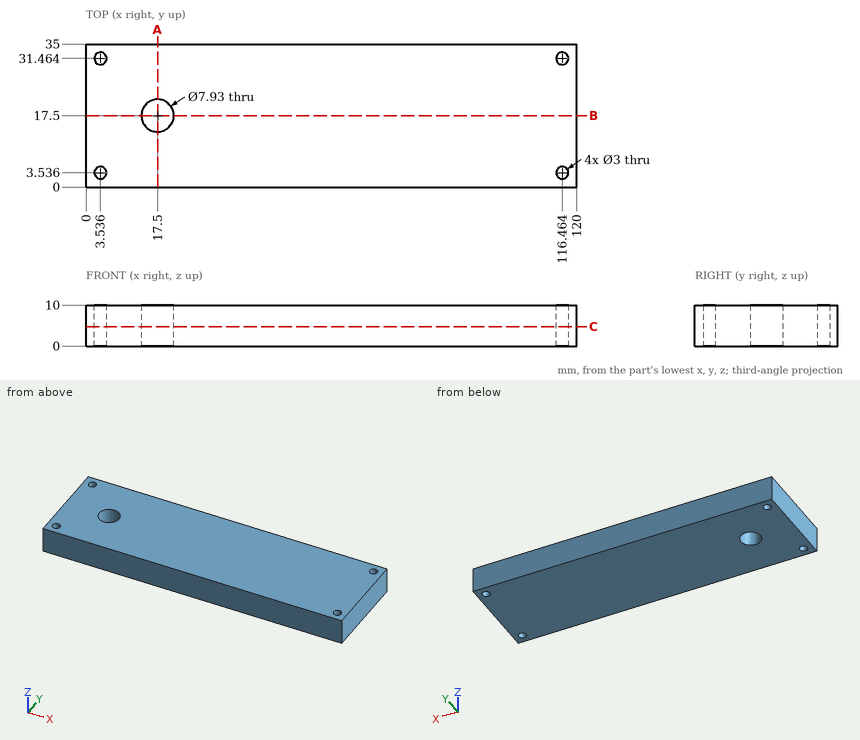
Verification items for this drawing (mm, ordinates from the low corner). Give positions to 0.01 mm unless a question says otherwise; leave off trailing zeros. Write each loop counter-clockwise with the first axis right and the second up, starting at its lowest first coordinate (ties: lowest second). Pieces come first, ordered by that corner, then holes. Notation, with made-up numbers: (13, 26) - (64, 26) arc R21 cw to (64, 33) - close; hole circle Ø3 at (47, 28.5). An arc over 180 degrees is marked (long way). Answer as a JSON object with one key per item and string values. Group by question number.
1) Sectioned sample at A-A (x = 17.5). Record the cut outline in (y, z) (1 decimal).
2) Sectioned sample at B-B (y = 17.5). Record the cut outline in (x, z) (1 decimal).
3) Sectioned sample at C-C (z = 4.75). Record the cut outline in (x, y) (1 decimal), then the cut area to 3 significant figures.
4) Thickness scan on probe 1 along Y at (x, z) = (17.5, 4) (1 decimal); probe 2 along X at (y, z) = (20.5, 4) (1 decimal); probe 3 along X at (y, z) = (21, 5) (1 decimal). Record the ranges inside material, lowest first. Write a range as from..to.
5) Depth check by flat-ended pin: P1, Ø2.5, axis at x = 116.46, y = 31.46, coming from the +Z side. Enter the tip coordinate at first touch or a pass-through.
Geometry results:
{
 "1": {"outline": "(0, 0) - (13.5, 0) - (13.5, 10) - (0, 10) - close; (21.5, 0) - (35, 0) - (35, 10) - (21.5, 10) - close"},
 "2": {"outline": "(0, 0) - (13.5, 0) - (13.5, 10) - (0, 10) - close; (21.5, 0) - (120, 0) - (120, 10) - (21.5, 10) - close"},
 "3": {"outline": "(0, 0) - (120, 0) - (120, 35) - (0, 35) - close; hole circle Ø3 at (3.5, 3.5); hole circle Ø3 at (3.5, 31.5); hole circle Ø7.9 at (17.5, 17.5); hole circle Ø3 at (116.5, 3.5); hole circle Ø3 at (116.5, 31.5)", "area": "4,120 mm^2"},
 "4": {"probe 1": "y = 0..13.5, 21.5..35", "probe 2": "x = 0..14.9, 20.1..120", "probe 3": "x = 0..15.6, 19.4..120"},
 "5": {"P1": "passes through"}
}
